Build history of the part. All positions in model axes, mm. A direction names the side the tool comes from. Round coordinates to 2 decimals unless told otherwise and drop trailing zeros. Order: outer loops, then holes, each group sorted by start corner. A loop starts at its lowest first (then second) coordinate and runs counter-clockwise, first axis right, second up. Notation, with made-up numbers: M 76.5,-20 L 132.5,-20 A34 ccw 132.5,18 Z; hole C 49,38.25 d1. An arc over 180 degrees is marked long. One line per question, with ' | ' between items. Start each with the question number.
from build123d import *

# Parameters (mm, degrees)
SKETCH1_R                        = 57.15
BOSS_EXTRUDE1_DEPTH              = 19.05
F_7_8_0_875_DIAMETER_HOLE1_D     = 22.225
F_7_8_0_875_DIAMETER_HOLE1_DEPTH = 6.35
F_7_8_0_875_DIAMETER_HOLE1_TIP   = 6.677063629
SKETCH4_R                        = 5.953125
CUT_EXTRUDE1_DEPTH               = 1
CUT_EXTRUDE1_DEPTH_BACK          = 20.05
ANNULUS_CHANNEL_R                = 31.75
ANNULUS_CHANNEL_DEPTH_DEPTH      = 5.334
SKETCH7_R                        = 38.735
SKETCH7_R_2                      = 35.56
CUT_EXTRUDE5_DEPTH               = 2.286
CIRPATTERN1_COUNT                = 6


with BuildPart() as part:
    # Sketch1 → Boss-Extrude1 (new body)
    with BuildSketch(Plane(origin=(0, 0, 0), x_dir=(1, 0, 0), z_dir=(0, 1, 0))):
        Circle(SKETCH1_R)
    extrude(amount=BOSS_EXTRUDE1_DEPTH)

    # 7/8 (0.875) Diameter Hole1
    with Locations(Plane(origin=(0, 19.05, 0), x_dir=(1, 0, 0), z_dir=(0, 1, 0))):
        with Locations((0, 0)):
            Hole(F_7_8_0_875_DIAMETER_HOLE1_D / 2, depth=F_7_8_0_875_DIAMETER_HOLE1_DEPTH)
            with Locations((0, 0, -(F_7_8_0_875_DIAMETER_HOLE1_DEPTH + F_7_8_0_875_DIAMETER_HOLE1_TIP / 2))):  # 118° drill point
                Cone(0, F_7_8_0_875_DIAMETER_HOLE1_D / 2, F_7_8_0_875_DIAMETER_HOLE1_TIP, mode=Mode.SUBTRACT)

    # Sketch4 → Cut-Extrude1 (cut, two sides)
    with BuildSketch(Plane(origin=(0, 19.05, 0), x_dir=(1, 0, 0), z_dir=(0, 1, 0))) as cut_extrude1_sk:
        Circle(SKETCH4_R)
    extrude(amount=CUT_EXTRUDE1_DEPTH, mode=Mode.SUBTRACT)
    extrude(cut_extrude1_sk.sketch, amount=-CUT_EXTRUDE1_DEPTH_BACK, mode=Mode.SUBTRACT)

    # Annulus Channel → Annulus Channel Depth (cut)
    with BuildSketch(Plane(origin=(0, 19.05, 0), x_dir=(1, 0, 0), z_dir=(0, 1, 0))):
        Circle(ANNULUS_CHANNEL_R)
        with BuildLine():
            Line((-10.649273743, 3.175), (-25.200781238, 3.175))
            ThreePointArc((-25.200781238, 3.175), (-12.7, 21.997045256), (9.850759962, 23.412016747))
            Line((9.850759962, 23.412016747), (2.575006214, 10.810041593))
            ThreePointArc((2.575006214, 10.810041593), (5.55625, 9.6237073), (8.074267528, 7.635041593))
            Line((8.074267528, 7.635041593), (15.350021276, 20.237016747))
            ThreePointArc((15.350021276, 20.237016747), (25.4, 0), (15.350021276, -20.237016747))
            Line((15.350021276, -20.237016747), (8.074267528, -7.635041593))
            ThreePointArc((8.074267528, -7.635041593), (5.55625, -9.6237073), (2.575006214, -10.810041593))
            Line((2.575006214, -10.810041593), (9.850759962, -23.412016747))
            ThreePointArc((9.850759962, -23.412016747), (-12.7, -21.997045256), (-25.200781238, -3.175))
            Line((-25.200781238, -3.175), (-10.649273743, -3.175))
            ThreePointArc((-10.649273743, -3.175), (-11.1125, 0), (-10.649273743, 3.175))
        make_face(mode=Mode.SUBTRACT)
    extrude(amount=-ANNULUS_CHANNEL_DEPTH_DEPTH, mode=Mode.SUBTRACT)

    # Sketch7 → Cut-Extrude5 (cut)
    with BuildSketch(Plane(origin=(0, 19.05, 0), x_dir=(1, 0, 0), z_dir=(0, 1, 0))):
        Circle(SKETCH7_R)
        Circle(SKETCH7_R_2, mode=Mode.SUBTRACT)
    extrude(amount=-CUT_EXTRUDE5_DEPTH, mode=Mode.SUBTRACT)

    # Sketch9 → 1/4-20 Tapped Hole1 (revolve, cut)
    with BuildSketch(Plane(origin=(0, 19.05, -45.72), x_dir=(0, 0, 1), z_dir=(1, 0, 0))):
        Polygon((0, 0), (0, 15.503816902), (2.5527, 13.97), (2.5527, 0.861971048), (3.302, 0), align=None)
    f_1_4_20_tapped_hole1 = revolve(axis=Axis((0, 25.4, -45.72), (0, -1, 0)), mode=Mode.SUBTRACT)

    # CirPattern1: 1/4-20 Tapped Hole1 ×6 about axis
    cirpattern1_axis = Axis((0, 0, 0), (0, 1, 0))
    for i in range(1, CIRPATTERN1_COUNT):
        add(f_1_4_20_tapped_hole1.rotate(cirpattern1_axis, i * 360 / CIRPATTERN1_COUNT), mode=Mode.SUBTRACT)


solid = part.part
Item 1: Two-plate mould, pull along Z, no slides. Class faces 1 (the face through (37, 19.05, 12)), 2 (the face through (6.264, 16.42, -17.199)): +Z half, -Z half, draft (parallel to the pull), parting line (faces both ways), or undercut.
Item 2: Wall check: line 1 along Z through (x, y) = (-1.5, 9); line 2 along X through (y, z) = (2.25, 0); line 3 along X through (y, z) = (12.25, 22.86). Give the ranges that are in metal, low to high. Write a range as [from, to].
Item 3: Cut at C-C on z = 33.5. Write the cut outline in (x, y).
Item 4: Cut at B-B on y = 2. Write the cut outline in (x, z), then the cut area to 3 significant figures.
Item 5: Cut at D-D on x = 17. Write the cut outline in (y, z).
Item 6: Tool access for faces 3 (the face through (-4.724, 4.867, 3.622)), 4 (the face through (-7.709, 17.923, 34.714)): list every direction of +Z, -Z, +X, -X, +Y, -Y with a clear straight run to the whole face (end or side of a thin tool).
Item 7: Flat gauge pins, fed straight in: pin 1 (2 mm diameter, centred on y = 14.5, z = -29.5, fed in from -X); pin 2 (4.5 mm diameter, centred on x = -21.5, y = 17, fed in from -Z); pin 3 (5 mm diameter, centred on y = 9, z = -39.5, fed in from +X); pin 4 (9.5 mm diameter, centred on x = 0, z = 0, fed in from -Y). Where does each tip first touch, or does it go through?
Results found:
1) face 1: draft | face 2: undercut
2) line 1: z = [-57.13, -47.79], [-43.65, -5.76], [5.76, 43.65], [47.79, 57.13] | line 2: x = [-57.15, -5.95], [5.95, 57.15] | line 3: x = [-52.38, -42.15], [-37.04, 37.04], [42.15, 52.38]
3) outline: M -46.3,0 L 46.3,0 L 46.3,19.05 L 19.45,19.05 L 19.45,16.76 L 11.93,16.76 L 11.93,19.05 L -11.93,19.05 L -11.93,16.76 L -19.45,16.76 L -19.45,19.05 L -46.3,19.05 Z
4) outline: C 0,0 d114.3; hole C 0,0 d11.91 | area: 10,100 mm^2
5) outline: M 0,-54.56 L 19.05,-54.56 L 19.05,-34.81 L 16.76,-34.81 L 16.76,-31.23 L 19.05,-31.23 L 19.05,-26.82 L 13.72,-26.82 L 13.72,-18.87 L 19.05,-18.87 L 19.05,18.87 L 13.72,18.87 L 13.72,26.82 L 19.05,26.82 L 19.05,31.23 L 16.76,31.23 L 16.76,34.81 L 19.05,34.81 L 19.05,54.56 L 0,54.56 Z
6) face 3: +Y, -Y | face 4: +Y
7) pin 1: stops at x = -49.54 | pin 2: stops at z = -53.81 | pin 3: stops at x = 43.56 | pin 4: passes through
